Autodesk Inventor part; units mm, degrees
ref_plane "YZ Plane" through (0, 0, 0) normal (1, 0, 0) x (0, 1, 0)
ref_plane "XZ Plane" through (0, 0, 0) normal (0, 1, 0) x (-1, 0, 0)
ref_plane "XY Plane" through (0, 0, 0) normal (0, 0, 1) x (1, 0, 0)
sketch "Sketch1" plane through (0, 0, 0) normal (0, 0, 1) x (1, 0, 0)
  line L0 (0, 0) -> (125.4125, 0)
  line L1 (125.4125, 0) -> (125.4125, 50.8)
  line L2 (125.4125, 50.8) -> (0, 50.8)
  line L3 (0, 50.8) -> (0, 0)
  dimension "d0" = 50.8
  dimension "d1" = 125.4125
extrude "Extrusion1" add sketch "Sketch1" along normal blind 6.35
sketch "Sketch2" plane through (0, 0, 6.35) normal (0, 0, 1) x (1, 0, 0)
  line L0 (0, 0) -> (0, 50.8)
  line L1 (125.4125, 50.8) -> (125.4125, 0)
  point P0 (25.4, 25.4)
  point P1 (114.3, 25.4)
  point P2 (0, 25.4)
  dimension "d4" = 25.4
  dimension "d5" = 11.1125
hole "Hole1" at (25.4, 25.4, 6.35) at (114.3, 25.4, 6.35) direction (0, 0, -1) diameter 7.62 end through all
sketch "Sketch3" plane through (0, 50.8, 0) normal (0, 1, 0) x (1, 0, 0)
  line L0 (0, -6.35) -> (125.4125, -6.35)
  line L1 (0, 0) -> (0, -6.35)
  line L2 (101.8247, -6.35) -> (106.5326, -56.3502)
  line L3 (106.5326, -56.3502) -> (55.9563, -61.1124)
  line L4 (55.9563, -61.1124) -> (50.8, -6.35)
  dimension "d13" = 50.8
  dimension "d14" = 50.8
  dimension "d15" = 54.7624
  dimension "d16" = 5.379
extrude "Extrusion2" add sketch "Sketch3" against normal up to surface (50.8 mm away)
sketch "Sketch4" plane through (106.5326, 0, 56.3502) normal (0.0937434, 0, 0.9955964) x (0.9955964, 0, -0.0937434)
  line L0 (-50.8, 50.8) -> (0, 50.8)
  line L1 (-50.8, 50.8) -> (-50.8, 0)
  line L2 (-43.18, 46.355) -> (-7.62, 46.355)
  line L3 (-4.445, 43.18) -> (-4.445, 7.62)
  line L4 (-7.62, 4.445) -> (-43.18, 4.445)
  line L5 (-46.355, 7.62) -> (-46.355, 43.18)
  arc A0 (-43.18, 46.355) -> (-46.355, 43.18) centre (-43.18, 43.18) ccw
  arc A1 (-46.355, 7.62) -> (-43.18, 4.445) centre (-43.18, 7.62) ccw
  arc A2 (-7.62, 4.445) -> (-4.445, 7.62) centre (-7.62, 7.62) ccw
  arc A3 (-4.445, 43.18) -> (-7.62, 46.355) centre (-7.62, 43.18) ccw
  point P0 (-100.781, 0)
  point P1 (-25.4, 46.355)
  point P2 (-25.4, 50.8)
  point P3 (-46.355, 25.4)
  point P4 (-50.8, 25.4)
  dimension "d19" = 3.175
  dimension "d20" = 4.445
  dimension "d21" = 4.445
extrude "Extrusion3" cut sketch "Sketch4" against normal up to surface surface through (62.7063, 25.4, 6.35) normal (0, 0, 1)
fillet "Fillet1" radius 6.35 4 edges at (53.3782, 50.8, 33.7312) (53.3782, 0, 33.7312) (104.1787, 50.8, 31.3501) (104.1787, 0, 31.3501)
hole "Hole2" at (78.8634, 50.8, 33.4432) direction (0, -1, 0) diameter 7.62 end through all
properties part number "frame bracket" material "Steel"
Geometry: final body of the model. Coordinates: model frame, mm. A direction names the side the tool comes from. Round coordinates to 2 decimals unless told otherwise and drop trailing zeros. Order: outer loops, then holes, each group sorted by start corner. A loop starts at its lowest first (then second) coordinate and runs counter-clockwise, first axis right, second up. Notation, with made-up numbers: (-6.75, 59.25) -> (24.25, 59.25) arc R33 ccw to (24.25, 88.25) -> close; hole circle Ø4 at (5.5, 50). An arc over 180 degrees is marked (long way). Put each result on its own line as item: value. Start each with the question number.
Q1. First-contact query: pin 1 (12.5 mm diameter, centred on x = 86.5, y = 20.5, fed in from +Z); pin 2 (10 mm diameter, centred on y = 21.5, z = 17, fed in from +X); pin 3 (12 mm diameter, centred on y = 18, z = 41.5, fed in from +X). Flat tips, straight axial feed; report the tip coordinate or a pass-through.
Q2. Reachability of faces 1 (the cylindrical face through (58.81, 45.45, 33.81)), 2 (the cylindrical face through (102.28, 1.81, 31.59)), 3 (the flat face through (53.414, 25.667, 34.115)), 4 (the flat face through (125.412, 25, 3)), 5 (the cylindrical face through (98.85, 45.4, 31.85)) from +Z, -Z, +X, -X, +Y, -Y: full face, straight path, thin tool, end or side. Return the list, or none.
Q3. Section B-B on y = 25.4. Return the cut outline in (x, z).
Q4. Section D-D on x = 14.5. Return the cut outline in (y, z).
Q5. Section C-C on y = 38. Return the cut outline in (x, z), and give its area (3 significant figures).
Q6. Pull-direction query (Z, two-part tool) for faces 6 (the flat face through (76, 0, 23)), 7 (the cylindrical face through (55.243, 1.811, 33.169)), 8 (the cylindrical face through (82.244, 48.546, 35.201)); classes: +Z half, -Z half, draft (parallel to the pull), parting line (faces both ways), or undercut.
Q7. Line query: probe 1 along X at (y, z) = (25, 1); probe 2 along Y at (x, z) = (80, 56.5) (3 decimals); probe 3 along Y at (x, z) = (114.3, 3.25). Output: solid intervals per line, ascending.
Q8. Section A-A on x = 114.3. Return the cut outline in (y, z).
Ans:
1. pin 1: stops at z = 6.35
1. pin 2: stops at x = 103.3
1. pin 3: stops at x = 105.7
2. face 1: none
2. face 2: +X, -Y
2. face 3: +Z, -X, +Y, -Y
2. face 4: +Z, -Z, +X, +Y, -Y
2. face 5: +Z
3. outline: (0, 0) -> (21.59, 0) -> (21.59, 6.35) -> (0, 6.35) -> close; (29.21, 0) -> (110.49, 0) -> (110.49, 6.35) -> (101.82, 6.35) -> (106.53, 56.35) -> (102.11, 56.77) -> (97.36, 6.35) -> (55.26, 6.35) -> (60.38, 60.7) -> (55.96, 61.11) -> (50.8, 6.35) -> (29.21, 6.35) -> close; (118.11, 0) -> (125.41, 0) -> (125.41, 6.35) -> (118.11, 6.35) -> close
4. outline: (0, 0) -> (50.8, 0) -> (50.8, 6.35) -> (0, 6.35) -> close
5. outline: (0, 0) -> (125.41, 0) -> (125.41, 6.35) -> (101.82, 6.35) -> (106.53, 56.35) -> (102.11, 56.77) -> (97.36, 6.35) -> (55.26, 6.35) -> (60.38, 60.7) -> (55.96, 61.11) -> (50.8, 6.35) -> (0, 6.35) -> close
5. area: 1,260 mm2
6. face 6: draft
6. face 7: +Z half
6. face 8: undercut
7. probe 1: x = 0 to 21.61, 29.19 to 110.51, 118.09 to 125.41
7. probe 2: y = 0 to 4.445, 46.355 to 50.8
7. probe 3: y = 0 to 21.59, 29.21 to 50.8
8. outline: (0, 0) -> (21.59, 0) -> (21.59, 6.35) -> (0, 6.35) -> close; (29.21, 0) -> (50.8, 0) -> (50.8, 6.35) -> (29.21, 6.35) -> close
